Design review of the part built by this model. Coordinates are the model's own, in mm. Face numbers are marked on the shaded views. A direction names the side the tool comes from. Coordinates: 2 decimals unless noted, no trailing zeros. Loops run counter-clockwise (first coordinate to the right, second up) from the corner with the lowest first, then second, coordinate; pieces in that order, holes last. Notation, with made-up numbers: (50.25, -28) -> (54.25, -28) arc R9 cw to (54.25, -12) -> close; hole circle Ø9 at (-12.5, -8). An arc over 180 degrees is marked (long way). Answer as a JSON object with one key per item and string values.
```python
from build123d import *

# Parameters (mm, degrees)
M4_TAPPED_HOLE1_D     = 3.3
M4_TAPPED_HOLE1_DEPTH = 5
M4_TAPPED_HOLE1_TIP   = 0.991420021
M3_TAPPED_HOLE1_D     = 2.5
M3_TAPPED_HOLE1_DEPTH = 3
M3_TAPPED_HOLE1_TIP   = 0.751075774
M3_TAPPED_HOLE2_D     = 2.5
M3_TAPPED_HOLE2_DEPTH = 3
M3_TAPPED_HOLE2_TIP   = 0.751075774


with BuildPart() as part:
    # Sketch1 → Revolve1 (revolve)
    with BuildSketch(Plane(origin=(0, 0, 0), x_dir=(0, 0, -1), z_dir=(1, 0, 0)), mode=Mode.PRIVATE) as revolve1_sk:
        Polygon((0, 0), (0, 18.5), (1.3, 18.5), (1.3, 24), (4.3, 24), (4.3, 49), (31.8, 49), (31.8, 35.5), (42.8, 35.5), (42.8, 0), align=None)
    revolve(revolve1_sk.sketch.rotate(Axis((0, 0, 42.770748728), (0, 0, -1)), 90), axis=Axis((0, 0, 42.770748728), (0, 0, -1)))

    # M4 Tapped Hole1
    with Locations(Plane.XY):
        with Locations((-14, 0), (-7, 12.124355653), (7, 12.124355653), (14, 0), (7, -12.124355653), (-7, -12.124355653)):
            Hole(M4_TAPPED_HOLE1_D / 2, depth=M4_TAPPED_HOLE1_DEPTH)
            with Locations((0, 0, -(M4_TAPPED_HOLE1_DEPTH + M4_TAPPED_HOLE1_TIP / 2))):  # 118° drill point
                Cone(0, M4_TAPPED_HOLE1_D / 2, M4_TAPPED_HOLE1_TIP, mode=Mode.SUBTRACT)

    # M3 Tapped Hole1
    with Locations(Plane.XY.offset(-4.3)):
        with Locations((-42.5, 0), (-30.0520382, 30.0520382), (0, 42.5), (30.0520382, 30.0520382), (42.5, 0), (30.0520382, -30.0520382), (0, -42.5), (-30.0520382, -30.0520382)):
            Hole(M3_TAPPED_HOLE1_D / 2, depth=M3_TAPPED_HOLE1_DEPTH)
            with Locations((0, 0, -(M3_TAPPED_HOLE1_DEPTH + M3_TAPPED_HOLE1_TIP / 2))):  # 118° drill point
                Cone(0, M3_TAPPED_HOLE1_D / 2, M3_TAPPED_HOLE1_TIP, mode=Mode.SUBTRACT)

    # M3 Tapped Hole2
    with Locations(Plane(origin=(0, 0, -31.8), x_dir=(-1, 0, 0), z_dir=(0, 0, -1))):
        with Locations((-42.5, 0), (-30.0520382, 30.0520382), (0, 42.5), (30.0520382, 30.0520382), (42.5, 0), (30.0520382, -30.0520382), (0, -42.5), (-30.0520382, -30.0520382)):
            Hole(M3_TAPPED_HOLE2_D / 2, depth=M3_TAPPED_HOLE2_DEPTH)
            with Locations((0, 0, -(M3_TAPPED_HOLE2_DEPTH + M3_TAPPED_HOLE2_TIP / 2))):  # 118° drill point
                Cone(0, M3_TAPPED_HOLE2_D / 2, M3_TAPPED_HOLE2_TIP, mode=Mode.SUBTRACT)


solid = part.part
```
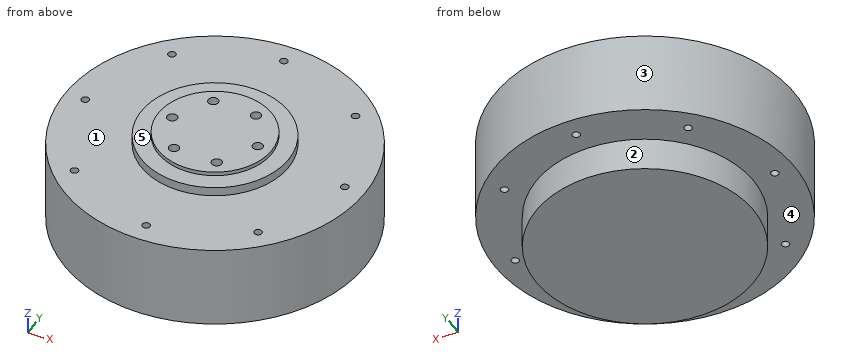
1) Clearance check with flat-ended pins moving along their axes: pin 1 Ø3 at (x, y) = (-30.05, 30.05) entering from +Z; pin 2 Ø4 at (y, z) = (-1, -36) entering from +X; pin 3 Ø3 at (x, y) = (37.5, 24) entering from -Z; pin 4 Ø4 at (y, z) = (-1.5, -14) entering from -X. State where each tip first meets the part, or that it passes through.
Completed:
{"pin 1": "z = -4.3", "pin 2": "x = 35.5", "pin 3": "z = -31.8", "pin 4": "x = -49"}
2) Add section C-C, the plane x = -20. Give the boundary of the cut face in (y, z).
Completed:
{"outline": "(-44.73, -31.8) -> (-29.33, -31.8) -> (-29.33, -42.8) -> (29.33, -42.8) -> (29.33, -31.8) -> (44.73, -31.8) -> (44.73, -4.3) -> (13.27, -4.3) -> (13.27, -1.3) -> (-13.27, -1.3) -> (-13.27, -4.3) -> (-44.73, -4.3) -> close"}
3) Wall thickness on probe 1 along Y at (x, z) = (0, -29.65); probe 2 along Y at (x, z) = (7, -3.3); probe 3 along Z at (x, y) = (-43.5, -4.5): over which ranges is each line inside the solid? List them lowest first.
Completed:
{"probe 1": "-49 to -43.75, -41.25 to 41.25, 43.75 to 49", "probe 2": "-22.96 to -13.77, -10.47 to 10.47, 13.77 to 22.96", "probe 3": "-31.8 to -4.3"}
4) For the marked faces 3, 4 and 5, list the 3-axis set-ups (+Z, -Z, +X, -X, +Y, -Y) from which the entire face can be reached by the end or side of a thin tool; tool diameter is ignored.
Completed:
{"face 3": "+Z, -Z", "face 4": "-Z", "face 5": "+Z"}
5) Add section A-A, the plane y = 32.5. Give the boundary of the cut face in (x, z).
Completed:
{"outline": "(-36.67, -31.8) -> (-14.28, -31.8) -> (-14.28, -42.8) -> (14.28, -42.8) -> (14.28, -31.8) -> (36.67, -31.8) -> (36.67, -4.3) -> (-36.67, -4.3) -> close"}
6) Add section B-B, the plane z = -26.5. Give the boundary of the cut face in (x, y), and give its area (3 significant figures).
Completed:
{"outline": "circle Ø98 at (0, 0)", "area": "7,540 mm²"}
7) The part is to be moulded in two halves that separate along X. For the marked faces 1 and 2, say which applies: pulls with the +X half, pulls with the -X half, needs draft (parallel to the pull), parting line crosses it, or undercut.
Completed:
{"face 1": "needs draft", "face 2": "parting line crosses it"}
8) Add section D-D, the plane y = -3. Give the boundary of the cut face in (x, z).
Completed:
{"outline": "(-48.91, -31.8) -> (-35.37, -31.8) -> (-35.37, -42.8) -> (35.37, -42.8) -> (35.37, -31.8) -> (48.91, -31.8) -> (48.91, -4.3) -> (23.81, -4.3) -> (23.81, -1.3) -> (18.26, -1.3) -> (18.26, 0) -> (-18.26, 0) -> (-18.26, -1.3) -> (-23.81, -1.3) -> (-23.81, -4.3) -> (-48.91, -4.3) -> close"}
